from build123d import *

# Parameters (mm, degrees)
BOSS_EXTRUDE1_DEPTH = 25


with BuildPart() as part:
    # Sketch1 → Boss-Extrude1 (new body)
    with BuildSketch(Plane.XY):
        with BuildLine():
            Line((-20, 0), (-20, -10))
            Line((-20, -10), (-10, -10))
            Line((-10, -10), (0, 0))
            ThreePointArc((0, 0), (-7.071067812, 2.928932188), (-10, 10))
            ThreePointArc((-10, 10), (-17.071067812, 7.071067812), (-20, 0))
        make_face()
    extrude(amount=BOSS_EXTRUDE1_DEPTH)


solid = part.part
Geometry check sheet. Reference: the model listing, model coordinates, mm. Give positions to 0.01 mm unless a question says otherwise; leave off trailing zeros. Order: outer loops, then holes, each group sorted by start corner. A loop starts at its lowest first (then second) coordinate and runs counter-clockwise, first axis right, second up. Notation, with made-up numbers: M 25.25,76 L 51.25,76 A17 ccw 51.25,81 Z; hole C -28,73.5 d7. An arc over 180 degrees is marked long. Use a Markdown table: item, result.
Item 1: Draft check along Y on faces 1 (the flat face through (-15, -10, 12)), 2 (the flat face through (-12, -2, 25)), 3 (the cylindrical face through (-16.99, 7.15, 12.32)). Enter one of: +Y half, -Y half, draft (parallel to the pull), parting line (faces both ways), or undercut.
Answers follow:
| item | result |
|---|---|
| face 1 | -Y half |
| face 2 | draft |
| face 3 | +Y half |
Item 2: Section check C-C (x = -18). Record the cut outline in (y, z).
Answers follow:
| item | result |
|---|---|
| outline | M -10,0 L 6,0 L 6,25 L -10,25 Z |
Item 3: Section check B-B (z = 9.5). Record the cut outline in (x, y).
Answers follow:
| item | result |
|---|---|
| outline | M -20,-10 L -10,-10 L 0,0 A10 cw -10,10 A10 ccw -20,0 Z |
Item 4: Section check A-A (y = -1.75). Record the cut outline in (x, z).
Answers follow:
| item | result |
|---|---|
| outline | M -20,0 L -1.75,0 L -1.75,25 L -20,25 Z |
Item 5: Material ranges on line 1 along X through (y, z) = (1, 8.25); line 2 along X through (y, z) = (-1, 14.5); line 3 along Y through (x, z) = (-5.5, 7.75), recorded low to high.
Answers follow:
| item | result |
|---|---|
| line 1 | x = -19.95 to -4.36 |
| line 2 | x = -20 to -1 |
| line 3 | y = -5.5 to 1.65 |
Item 6: Depth check by flat-ended pin: P1, Ø3, axis at x = -7.5, z = 8, coming from the +Y side. Enter the tip coordinate at first touch or a pass-through.
Answers follow:
| item | result |
|---|---|
| P1 | stops at y = 5.64 |
